Geometry check sheet. Reference: the model listing, model coordinates, mm. Round coordinates to 2 decimals unless told otherwise and drop trailing zeros. Loops run counter-clockwise (first coordinate to the right, second up) from the corner with the lowest first, then second, coordinate; pieces in that order, holes last. Notation, with made-up numbers: (-3, 42) - (17, 42) arc R5 cw to (17, 51) - close; hole circle Ø4 at (38, 47). An arc over 180 degrees is marked (long way). Write item = value, one per line.
```python
from build123d import *

# Parameters (mm, degrees)
SKETCH1_R           = 4
SKETCH1_R_2         = 3
BOSS_EXTRUDE1_DEPTH = 3.175


with BuildPart() as part:
    # Sketch1 → Boss-Extrude1 (new body)
    with BuildSketch(Plane(origin=(0, 0, 0), x_dir=(1, 0, 0), z_dir=(0, 1, 0))):
        with BuildLine():
            Line((-42.06875, 8.658790241), (-10.583333333, 23.090107309))
            ThreePointArc((-10.583333333, 23.090107309), (0, 25.4), (10.583333333, 23.090107309))
            Line((10.583333333, 23.090107309), (42.06875, 8.658790241))
            ThreePointArc((42.06875, 8.658790241), (47.625, 0), (42.06875, -8.658790241))
            Line((42.06875, -8.658790241), (10.583333333, -23.090107309))
            ThreePointArc((10.583333333, -23.090107309), (0, -25.4), (-10.583333333, -23.090107309))
            Line((-10.583333333, -23.090107309), (-42.06875, -8.658790241))
            ThreePointArc((-42.06875, -8.658790241), (-47.625, 0), (-42.06875, 8.658790241))
        make_face()
        with Locations((-38.1, 0)):
            Circle(SKETCH1_R, mode=Mode.SUBTRACT)
        with Locations((38.1, 0)):
            Circle(SKETCH1_R, mode=Mode.SUBTRACT)
        with Locations((6.35, 0)):
            Circle(SKETCH1_R_2, mode=Mode.SUBTRACT)
        with Locations((-6.35, 0)):
            Circle(SKETCH1_R_2, mode=Mode.SUBTRACT)
    extrude(amount=-BOSS_EXTRUDE1_DEPTH)


solid = part.part
```
(1) Section check C-C (x = -39). Enter the section's corners in (y, z) (3 decimals), then the cut area to 3 significant figures.
Answers follow:
outline = (-3.175, -10.065) - (0, -10.065) - (0, -3.897) - (-3.175, -3.897) - close; (-3.175, 3.897) - (0, 3.897) - (0, 10.065) - (-3.175, 10.065) - close
area = 39.2 mm²
(2) Scan lines: L1, parallel to X at y = -1.7, z = 0 (3 decimals); L2, parallel to X at y = -1.05, z = 3.5; L3, parallel to Z at x = -6.35, y = -2.35. Record each from-to range of solid material in increasing order. Write a range as [from, to].
Answers follow:
L1 = [-47.625, -42.1], [-34.1, -9.35], [-3.35, 3.35], [9.35, 34.1], [42.1, 47.625]
L2 = [-46.96, -40.04], [-36.16, 36.16], [40.04, 46.96]
L3 = [-24.59, -3], [3, 24.59]
(3) Section check A-A (y = -1.35). Enter the section's corners in (x, z) (3 decimals).
Answers follow:
outline = (-42.069, -8.659) - (-10.583, -23.09) arc R25.4 ccw to (10.583, -23.09) - (42.069, -8.659) arc R9.525 ccw to (42.069, 8.659) - (10.583, 23.09) arc R25.4 ccw to (-10.583, 23.09) - (-42.069, 8.659) arc R9.525 ccw to start; hole circle Ø8 at (-38.1, 0); hole circle Ø6 at (-6.35, 0); hole circle Ø6 at (6.35, 0); hole circle Ø8 at (38.1, 0)
(4) Gauge pin test, flat ends, axial feed: pin 1 (5 mm diameter, centred on x = -38.1, z = 0, fed in from -Y); pin 2 (1.5 mm diameter, centred on y = -2, z = -4, fed in from -X); pin 3 (1.5 mm diameter, centred on x = 19, y = -2, fed in from +Z). Record the tip position at first contact, or that the pin passes through.
Answers follow:
pin_1 = through
pin_2 = -47.05
pin_3 = 19.58
(5) Section check D-D (x = 38.1). Enter the section's corners in (y, z) (3 decimals).
Answers follow:
outline = (-3.175, -10.478) - (0, -10.478) - (0, -4) - (-3.175, -4) - close; (-3.175, 4) - (0, 4) - (0, 10.478) - (-3.175, 10.478) - close
(6) Mould release check, pull along Z, two halves, no side actions. Record for faces 1 (the cylindrical face through (0.2, -1.6, 25.4)), 2 (the cylindrical face through (-34.405, -1.565, 1.532)), 3 (the cylindrical face through (3.969, -1.565, 1.825)), 4 (the flat face through (1, -3.175, 0)): pulls with the +Z half, pulls with the -Z half, needs draft (parallel to the pull), parting line crosses it, or undercut.
Answers follow:
face_1 = pulls with the +Z half
face_2 = undercut
face_3 = undercut
face_4 = needs draft
(7) Section check B-B (z = 0). Enter the section's corners in (x, y) (3 decimals), then the cut area to 3 significant figures.
Answers follow:
outline = (-47.625, -3.175) - (-42.1, -3.175) - (-42.1, 0) - (-47.625, 0) - close; (-34.1, -3.175) - (-9.35, -3.175) - (-9.35, 0) - (-34.1, 0) - close; (-3.35, -3.175) - (3.35, -3.175) - (3.35, 0) - (-3.35, 0) - close; (9.35, -3.175) - (34.1, -3.175) - (34.1, 0) - (9.35, 0) - close; (42.1, -3.175) - (47.625, -3.175) - (47.625, 0) - (42.1, 0) - close
area = 214 mm²
